Geometry: final body of the model. Coordinates: model frame, mm. A direction names the side the tool comes from. Give positions to 0.01 mm unless a question says otherwise; leave off trailing zeros. Write each loop counter-clockwise with the first axis right and the second up, starting at its lowest first coordinate (ties: lowest second). Pieces come first, ordered by that corner, then holes. Notation, with made-up numbers: M -27.75,-21 L 28.25,-21 A24 cw 28.25,-7 Z; hole C 4.25,33.5 d7. An arc over 180 degrees is marked long. Use a Markdown table: item, result. Add a question column.
1) Section A-A on x = -10. Return the cut outline in (y, z), then the cut area to 3 significant figures.
2) Line query: line 1 (X direction, y = -13.05, z = 0); line 2 (Z direction, x = -15, y = 15); line 3 (X direction, y = 14.25, z = 0). Output: solid intervals per line, ascending.
3) Set-up query: faces 1 (the cylindrical face through (4.6, -26.8, -1.6)), 2 (the flat face through (-16, 0, 2)), 3 (the cylindrical face through (5.99, 27.44, -6.24)). Return all of +Z, -Z, +X, -X, +Y, -Y with unobstructed straight access to the full face (end or side cutting, diameter ignored); none if empty.
4) Section D-D on y = 25.5. Return the cut outline in (x, z), then the cut area to 3 significant figures.
5) Section C-C on x = 13. Return the cut outline in (y, z).
6) Section B-B on y = -2. Return the cut outline in (x, z), then the cut area to 3 significant figures.
7) Draft query along X for faces 4 (the flat face through (1, 31, 2)), 5 (the flat face through (-19, 16, 0)), 6 (the cylindrical face through (-17.19, 15.07, -4.6)). Return one class per face: +X half, -X half, draft (parallel to the pull), parting line (faces both ways), or undercut.
8) Pin query (flat end, axial travel): pin 1 (8 mm diameter, centred on y = -12.5, z = -6.5, fed in from -X); pin 2 (4 mm diameter, centred on y = 5, z = 5, fed in from +X); pin 3 (1.2 mm diameter, centred on x = -0.5, z = -1, fed in from +Y). Return the tip coordinate at first contact, or that it passes through.
```python
from build123d import *

# Parameters (mm, degrees)
BOSS_EXTRUDE1_DEPTH      = 10
CUT_EXTRUDE1_DEPTH       = 67.219333
CUT_EXTRUDE2_DEPTH       = 2
M3_TAPPED_HOLE1_D        = 2.5
M3_TAPPED_HOLE1_DEPTH    = 9
M3_TAPPED_HOLE1_TIP      = 0.751076
SKETCH6_R                = 2.5
CUT_EXTRUDE3_DEPTH       = 44.185646
SKETCH7_R                = 4
CUT_EXTRUDE4_DEPTH       = 53.191953
CHAMFER1_SIZE            = 1
HOLE1_START              = 2
HOLE1_OUTLINE_R          = 2
HOLE1_DEPTH              = 28
HOLE1_START_2            = -17
HOLE1_2_OUTLINE_R        = 1.25
HOLE1_2_DEPTH            = 19
CUT_EXTRUDE5_REACH       = 54.192
CUT_EXTRUDE5_END_RADIUS  = 7
SKETCH10_R               = 1.6
CUT_EXTRUDE6_START       = -6.35617
CUT_EXTRUDE6_OUTLINE_R   = 1.65
CUT_EXTRUDE6_DEPTH       = 6.35617
CUT_EXTRUDE6_START_2     = -17.834937
CUT_EXTRUDE6_2_OUTLINE_R = 1.25
CUT_EXTRUDE6_2_DEPTH     = 11.478767


with BuildPart() as part:
    # Sketch2 → Boss-Extrude1 (new, symmetric)
    with BuildSketch(Plane.XY):
        Polygon((0, 0), (-19, 0), (-19, 32), (9, 32), (21, -6), (21, -30), (0, -30), align=None)
    extrude(amount=BOSS_EXTRUDE1_DEPTH, both=True)

    # Sketch3 → Cut-Extrude1 (cut, through all)
    with BuildSketch(Plane(origin=(0, 32, 0), x_dir=(1, 0, 0), z_dir=(0, 1, 0))):
        with BuildLine():
            ThreePointArc((-2.291796, 2), (-10.010587, 6.926667), (-16, 0))
            Line((-16, 0), (-2, 0))
            ThreePointArc((-2, 0), (-2.073333, 1.010587), (-2.291796, 2))
        make_face()
        with BuildLine():
            Line((-2, 0), (-16, 0))
            ThreePointArc((-16, 0), (-10.010587, -6.926667), (-2.291796, -2))
            ThreePointArc((-2.291796, -2), (-2.073333, -1.010587), (-2, 0))
        make_face()
    extrude(amount=-CUT_EXTRUDE1_DEPTH, mode=Mode.SUBTRACT)

    # Sketch3<3> → Cut-Extrude2 (cut)
    with BuildSketch(Plane(origin=(0, 32, 0), x_dir=(1, 0, 0), z_dir=(0, 1, 0))):
        with BuildLine():
            ThreePointArc((-2.291796, 2), (-2.073333, 1.010587), (-2, 0))
            Line((-2, 0), (3, 0))
            ThreePointArc((3, 0), (3.585786, 1.414214), (5, 2))
            Line((5, 2), (-2.291796, 2))
        make_face()
        with BuildLine():
            Line((3, 0), (-2, 0))
            ThreePointArc((-2, 0), (-2.073333, -1.010587), (-2.291796, -2))
            Line((-2.291796, -2), (5, -2))
            ThreePointArc((5, -2), (3.585786, -1.414214), (3, 0))
        make_face()
        with BuildLine():
            ThreePointArc((5, 2), (3.585786, 1.414214), (3, 0))
            Line((3, 0), (7, 0))
            ThreePointArc((7, 0), (6.414214, 1.414214), (5, 2))
        make_face()
        with BuildLine():
            Line((7, 0), (3, 0))
            ThreePointArc((3, 0), (3.585786, -1.414214), (5, -2))
            ThreePointArc((5, -2), (6.414214, -1.414214), (7, 0))
        make_face()
    extrude(amount=-CUT_EXTRUDE2_DEPTH, mode=Mode.SUBTRACT)

    # M3 Tapped Hole1
    with Locations(Plane(origin=(0, 32, 0), x_dir=(1, 0, 0), z_dir=(0, 1, 0))):
        with Locations((-16, 7), (-16, -7), (5, -7), (5, 7)):
            Hole(M3_TAPPED_HOLE1_D / 2, depth=M3_TAPPED_HOLE1_DEPTH)
            with Locations((0, 0, -(M3_TAPPED_HOLE1_DEPTH + M3_TAPPED_HOLE1_TIP / 2))):  # 118° drill point
                Cone(0, M3_TAPPED_HOLE1_D / 2, M3_TAPPED_HOLE1_TIP, mode=Mode.SUBTRACT)

    # Sketch6 → Cut-Extrude3 (cut, through all)
    with BuildSketch(Plane.XY.offset(10)):
        with Locations((13, -10)):
            Circle(SKETCH6_R)
    extrude(amount=-CUT_EXTRUDE3_DEPTH, mode=Mode.SUBTRACT)

    # Sketch7 → Cut-Extrude4 (cut, through all)
    with BuildSketch(Plane(origin=(21, 0, 0), x_dir=(0, 0, -1), z_dir=(1, 0, 0))):
        with Locations((0, -20)):
            Circle(SKETCH7_R)
    extrude(amount=-CUT_EXTRUDE4_DEPTH, mode=Mode.SUBTRACT)

    # Chamfer1
    chamfer1_edges = [part.edges().sort_by_distance(p)[0] for p in [
        (21, -20, 4),
    ]]
    chamfer(chamfer1_edges, length=CHAMFER1_SIZE)

    # Hole1: read off the stored shape, not the designer's step
    # Hole1 outline → Hole1 (cut)
    with BuildSketch(Plane(origin=(0, 0, 0), x_dir=(1, 0, 0), z_dir=(0, 1, 0)).offset(HOLE1_START)):
        with Locations((5, 0)):
            Circle(HOLE1_OUTLINE_R)
    extrude(amount=HOLE1_DEPTH, mode=Mode.SUBTRACT)

    # Hole1 2 outline → Hole1 2 (cut)
    with BuildSketch(Plane(origin=(0, 0, 0), x_dir=(1, 0, 0), z_dir=(0, 1, 0)).offset(HOLE1_START_2)):
        with Locations((5, 0)):
            Circle(HOLE1_2_OUTLINE_R)
    extrude(amount=HOLE1_2_DEPTH, mode=Mode.SUBTRACT)

    # Cut-Extrude5: up to this cylinder (the profile starts outside it)
    cut_extrude5_end = Plane(origin=(-9, 15, 0), z_dir=(0, 1, 0)) * Cylinder(CUT_EXTRUDE5_END_RADIUS, 123.384, mode=Mode.PRIVATE)
    # Sketch10 → Cut-Extrude5 (cut, up to the surface)
    with BuildSketch(Plane.ZY.offset(19), mode=Mode.PRIVATE) as cut_extrude5_sk1:
        with Locations((-3, 15)):
            Circle(SKETCH10_R)
    cut_extrude5_tool1 = extrude(cut_extrude5_sk1.sketch, amount=-CUT_EXTRUDE5_REACH, mode=Mode.PRIVATE) - cut_extrude5_end
    add(cut_extrude5_tool1.solids().sort_by_distance((-19, 15, -3))[0], mode=Mode.SUBTRACT)
    # Sketch10 → Cut-Extrude5 (cut, up to the surface)
    with BuildSketch(Plane.ZY.offset(19), mode=Mode.PRIVATE) as cut_extrude5_sk2:
        with Locations((3, 15)):
            Circle(SKETCH10_R)
    cut_extrude5_tool2 = extrude(cut_extrude5_sk2.sketch, amount=-CUT_EXTRUDE5_REACH, mode=Mode.PRIVATE) - cut_extrude5_end
    add(cut_extrude5_tool2.solids().sort_by_distance((-19, 15, 3))[0], mode=Mode.SUBTRACT)

    # Cut-Extrude6: read off the stored shape, not the designer's step
    # Cut-Extrude6 outline → Cut-Extrude6 (cut)
    with BuildSketch(Plane.XZ.offset(30).offset(CUT_EXTRUDE6_START)):
        with Locations((5, 0)):
            Circle(CUT_EXTRUDE6_OUTLINE_R)
        with Locations((13, 0)):
            Circle(CUT_EXTRUDE6_OUTLINE_R)
    extrude(amount=CUT_EXTRUDE6_DEPTH, mode=Mode.SUBTRACT)

    # Cut-Extrude6 2 outline → Cut-Extrude6 2 (cut)
    with BuildSketch(Plane.XZ.offset(30).offset(CUT_EXTRUDE6_START_2)):
        with Locations((13, 0)):
            Circle(CUT_EXTRUDE6_2_OUTLINE_R)
    extrude(amount=CUT_EXTRUDE6_2_DEPTH, mode=Mode.SUBTRACT)


solid = part.part
```
Found:
| question | item | result |
|---|---|---|
| 1 | outline | M 0,-10 L 32,-10 L 32,-6.93 L 0,-6.93 Z; M 0,6.93 L 32,6.93 L 32,10 L 0,10 Z |
| 1 | area | 197 mm² |
| 2 | line 1 | 0 to 3.75, 6.25 to 11.75, 14.25 to 21 |
| 2 | line 2 | -10 to -4.6, 4.6 to 10 |
| 2 | line 3 | -19 to -16, -2 to 3, 7 to 14.61 |
| 3 | face 1 | -Y |
| 3 | face 2 | +Z, -Z, -X, -Y |
| 3 | face 3 | +Y |
| 4 | outline | M -19,-10 L 11.05,-10 L 11.05,10 L -19,10 Z; hole C -16,-7 d2.5; hole C -16,7 d2.5; hole M -2.29,-2 A7 ccw -2,0 A7 ccw -2.29,2 A7 ccw long Z; hole C 5,0 d4; hole C 5,-7 d2.5; hole C 5,7 d2.5 |
| 4 | area | 415 mm² |
| 5 | outline | M -30,-10 L -12.5,-10 L -12.5,-1.25 L -16.2,-1.25 A4 cw -23.64,-1.65 L -30,-1.65 Z; M -30,1.65 L -23.64,1.65 A4 cw -16.2,1.25 L -12.5,1.25 L -12.5,10 L -30,10 Z; M -7.5,-10 L 19.33,-10 L 19.33,10 L -7.5,10 Z |
| 6 | outline | M 0,-10 L 19.74,-10 L 19.74,10 L 0,10 Z; hole C 5,0 d2.5 |
| 6 | area | 390 mm² |
| 7 | face 4 | undercut |
| 7 | face 5 | -X half |
| 7 | face 6 | draft |
| 8 | pin 1 | x = 0 |
| 8 | pin 2 | x = 18.16 |
| 8 | pin 3 | y = 30 |
